Design review of the part shown in the three views and the two pictorial views. Dimensions are in mm from the part's minimum x, y and z. Give positions to 0.01 mm unless a question says otherwise; leave off trailing zeros. Loops run counter-clockwise (first coordinate to the right, second up) from the corner with the lowest first, then second, coordinate; pieces in that order, holes last.
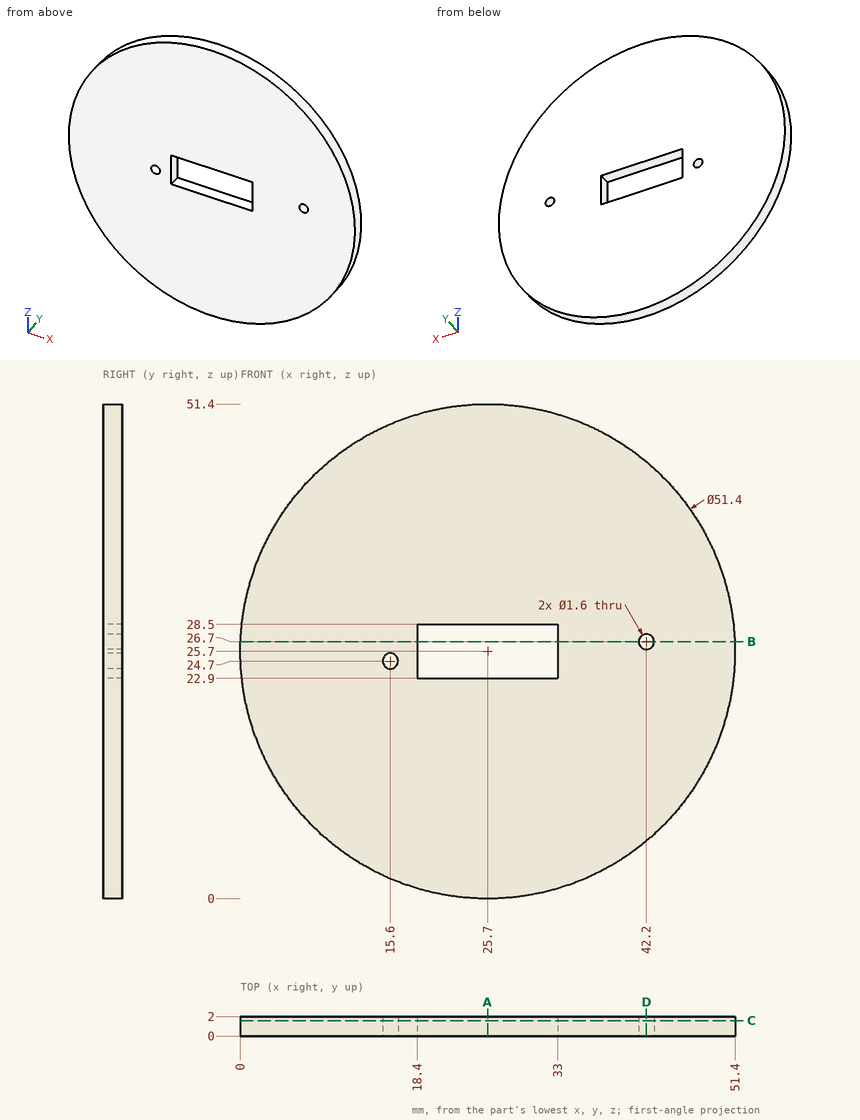
Q1. Wall thickness on line 1 (X direction, y = 1.1, z = 24.7); line 2 (X direction, y = 0.85, z = 26.7); line 3 (Z direction, x = 31, y = 1.7): over which ranges is each line inside the solid? List them lowest first.
Results:
line 1: x = 0.02 to 14.8, 16.4 to 18.4, 33 to 51.38
line 2: x = 0.02 to 18.4, 33 to 41.4, 43 to 51.38
line 3: z = 0.55 to 22.9, 28.5 to 50.85
Q2. Take a section at B-B (z = 26.7). Give the boundary of the cut face in (x, y).
Results:
outline: (0.02, 0) - (18.4, 0) - (18.4, 2) - (0.02, 2) - close; (33, 0) - (41.4, 0) - (41.4, 2) - (33, 2) - close; (43, 0) - (51.38, 0) - (51.38, 2) - (43, 2) - close
Q3. Take a section at C-C (y = 1.6). Give the boundary of the cut face in (x, z), plus the area to 3 significant figures.
Results:
outline: circle Ø51.4 at (25.7, 25.7); hole circle Ø1.6 at (15.6, 24.7); hole (18.4, 22.9) - (33, 22.9) - (33, 28.5) - (18.4, 28.5) - close; hole circle Ø1.6 at (42.2, 26.7)
area: 1,990 mm2
Q4. Take a section at A-A (x = 25.7). Give the boundary of the cut face in (y, z), plus the area to 3 significant figures.
Results:
outline: (0, 0) - (2, 0) - (2, 22.9) - (0, 22.9) - close; (0, 28.5) - (2, 28.5) - (2, 51.4) - (0, 51.4) - close
area: 91.6 mm2
Q5. Insertion check: pin 1 (1 mm diameter, centred on x = 17.5, z = 39.5, fed in from -Y); pin 2 (1.3 mm diameter, centred on x = 42.2, z = 26.7, fed in from -Y); pin 3 (0.6 mm diameter, centred on y = 1, z = 26.5, fed in from -X); pin 4 (0.6 mm diameter, centred on x = 23, y = 1.5, fed in from +Z). Each pin has a flat end and moves straight along its axis. Give the tip position at first contact, or say it passes through.
Results:
pin 1: stops at y = 0
pin 2: passes through
pin 3: stops at x = 0
pin 4: stops at z = 51.29
Q6. Take a section at D-D (x = 42.2). Give the boundary of the cut face in (y, z).
Results:
outline: (0, 6) - (2, 6) - (2, 25.9) - (0, 25.9) - close; (0, 27.5) - (2, 27.5) - (2, 45.4) - (0, 45.4) - close
